Input: part model. Units: mm. Frame: model coordinates. A direction names the side the tool comes from. Round coordinates to 2 decimals unless told otherwise and drop trailing zeros. Write each loop counter-clockwise with the first axis right and the second up, starting at its lowest first coordinate (ties: lowest second). Pieces come first, ordered by that corner, then holes. Notation, with made-up numbers: M 24.5,46.5 L 76.5,46.5 A18 cw 76.5,73.5 Z; hole C 3.25,-37 d8. An arc over 180 degrees is marked long. Write each question's results on one line, items separated by ' | '. Start each with the question number.
```python
from build123d import *

# Parameters (mm, degrees)
BOSS_EXTRUDE1_DEPTH  = 4
CUT_EXTRUDE1_DEPTH   = 10
M3_CLEARANCE_HOLE3_D = 3.4
M3_CLEARANCE_HOLE4_D = 3.4


with BuildPart() as part:
    # Sketch1 → Boss-Extrude1 (new body)
    with BuildSketch(Plane(origin=(0, 0, 0), x_dir=(1, 0, 0), z_dir=(0, 1, 0))):
        with BuildLine():
            Line((-9.515488572, -74.994808418), (9.515488572, -74.994808418))
            ThreePointArc((9.515488572, -74.994808418), (13.049333225, -73.843719838), (15.227255138, -70.832122406))
            Line((15.227255138, -70.832122406), (21.674585029, -50.788926983))
            ThreePointArc((21.674585029, -50.788926983), (21.904821248, -49.783840665), (21.959569126, -48.754175722))
            Line((21.959569126, -48.754175722), (20.905492982, -16.738783097))
            ThreePointArc((20.905492982, -16.738783097), (20.516685602, -14.802919609), (19.520547525, -13.098088957))
            Line((19.520547525, -13.098088957), (13, -5.263157895))
            Line((13, -5.263157895), (13, 5.263157895))
            Line((13, 5.263157895), (19.670378922, 13.278122714))
            ThreePointArc((19.670378922, 13.278122714), (20.587655893, 14.78617896), (21.026416806, 16.495892253))
            Line((21.026416806, 16.495892253), (23.354507229, 38.891979018))
            ThreePointArc((23.354507229, 38.891979018), (23.340591043, 40.254469199), (23.019622055, 41.578686728))
            Line((23.019622055, 41.578686728), (18.764127525, 53.179369038))
            ThreePointArc((18.764127525, 53.179369038), (16.566422509, 56.032274923), (13.131169609, 57.113023201))
            Line((13.131169609, 57.113023201), (-14.108422678, 57.113023201))
            ThreePointArc((-14.108422678, 57.113023201), (-17.566572488, 56.016205829), (-19.760402704, 53.126756496))
            Line((-19.760402704, 53.126756496), (-23.659003651, 42.184485876))
            ThreePointArc((-23.659003651, 42.184485876), (-23.973087581, 40.807997325), (-23.956822357, 39.396223658))
            Line((-23.956822357, 39.396223658), (-20.971772171, 16.465578606))
            ThreePointArc((-20.971772171, 16.465578606), (-20.532623688, 14.866769408), (-19.672669362, 13.44919373))
            Line((-19.672669362, 13.44919373), (-13, 5.263157895))
            Line((-13, 5.263157895), (-13, -5.263157895))
            Line((-13, -5.263157895), (-19.456827239, -13.021524214))
            ThreePointArc((-19.456827239, -13.021524214), (-20.441610734, -14.696742104), (-20.839350394, -16.598834814))
            Line((-20.839350394, -16.598834814), (-22.202521241, -47.927982232))
            ThreePointArc((-22.202521241, -47.927982232), (-22.154511659, -48.989610746), (-21.919959446, -50.026117032))
            Line((-21.919959446, -50.026117032), (-15.227255138, -70.832122406))
            ThreePointArc((-15.227255138, -70.832122406), (-13.049333225, -73.843719838), (-9.515488572, -74.994808418))
        make_face()
    extrude(amount=BOSS_EXTRUDE1_DEPTH)

    # Sketch6 → Cut-Extrude1 (cut)
    with BuildSketch(Plane(origin=(0, 4, 0), x_dir=(1, 0, 0), z_dir=(0, 1, 0))):
        Polygon((-10.921572875, 24.5), (10.921572875, 24.5), (0, 35.421572875), align=None)
        Polygon((-7.79159133, -53.303689334), (7.79159133, -53.303689334), (0, -56.489348074), align=None)
        Polygon((-13.076324897, -55.464397842), (-13.076324897, -61.835715323), (-5.284733567, -58.650056583), align=None)
        Polygon((13.75, 27.328427125), (2.828427125, 38.25), (13.75, 49.171572875), align=None)
        Polygon((-13.5, -29.271972435), (-3.109490994, -38), (-13.5, -46.728027565), align=None)
        Polygon((-10.104794721, -49.1), (0, -40.611972435), (10.104794721, -49.1), align=None)
        Polygon((-7.79159133, -63.996423832), (7.79159133, -63.996423832), (0, -60.810765091), align=None)
        Polygon((-13.75, 27.328427125), (-2.828427125, 38.25), (-13.75, 49.171572875), align=None)
        Polygon((13.076324897, -55.464397842), (13.076324897, -61.835715323), (5.284733567, -58.650056583), align=None)
        Polygon((0, 41.078427125), (10.921572875, 52), (-10.921572875, 52), align=None)
        Polygon((-10.104794721, -26.9), (10.104794721, -26.9), (0, -35.388027565), align=None)
        Polygon((3.109490994, -38), (13.5, -29.271972435), (13.5, -46.728027565), align=None)
    extrude(amount=-CUT_EXTRUDE1_DEPTH, mode=Mode.SUBTRACT)

    # M3 Clearance Hole3 (through all)
    with Locations(Plane(origin=(0, 4, 0), x_dir=(1, 0, 0), z_dir=(0, 1, 0))):
        with Locations((7.62, -69.497474683), (-7.62, -69.497474683), (-26.177409906, -26.177409906), (26.177409906, -26.177409906), (26.177409906, 26.177409906), (-26.177409906, 26.177409906), (-15, -25.4), (-15.25, 23), (-15.25, 53.5), (15.25, 53.5), (15.25, 23), (-15, -50.6), (15, -50.6), (15, -25.4), (20, 38.25), (-20, 38.25)):
            Hole(M3_CLEARANCE_HOLE3_D / 2)

    # M3 Clearance Hole4 (through all)
    with Locations(Plane(origin=(0, 4, 0), x_dir=(1, 0, 0), z_dir=(0, 1, 0))):
        with Locations((-10.606601718, 10.606601718), (-16.263455967, 16.263455967), (10.606601718, 10.606601718), (16.263455967, 16.263455967), (16.263455967, -16.263455967), (10.606601718, -10.606601718), (-10.606601718, -10.606601718), (-16.263455967, -16.263455967)):
            Hole(M3_CLEARANCE_HOLE4_D / 2)


solid = part.part
```
1. Access query for faces 4 (the face through (-20.43, 1.97, 14.67)), 5 (the face through (-8.377, 2.028, 33.575)), 6 (the face through (16.288, 1.972, -9.215)). Directions: +Z, -Z, +X, -X, +Y, -Y. A direction counts if a zero-diameter tool reaches every point of the face in a straight line with its end or side. Return the directions, or none.
2. Draft query along Z for faces 1 (the face through (-13.092, 1.972, 73.812)), 2 (the face through (-1, 0, 8)), 3 (the face through (-13.5, 2, 38)). Return one class per face: +Z half, -Z half, draft (parallel to the pull), parting line (faces both ways), or undercut.
3. Cut plane C-C on y = 2.25. Give the number of separate pieces and of enclosed holes in the cut face, and give its area (3 significant figures).
4. Contact query for flat-ended pins moving along their axis: P1, Ø2, axis at y = 2.5, z = -0.5, coming from the +X side; P2, Ø5.5, axis at x = 15, z = 25.4, coming from the -Y side; P3, Ø2.5, axis at x = -7.62, z = 69.5, coming from the +Y side; P4, Ø1, axis at y = 3, z = 28.5, coming from the -X side. Output: stop coordinate, or through.
5. Cut plane B-B on z = 25.4. Output: boundary loops of the cut face in (x, y), and give its area (3 significant figures).
6. Line query: L1, parallel to X at y = 1.25, z = 25.4; L2, parallel to X at y = 0.8, z = -43; L3, parallel to X at y = 2.75, z = -38.25. Output: solid intervals per line, ascending. Write a range as from..to.
7. Cut plane A-A on z = -23. Output: boundary loops of the cut face in (x, y), and give its area (3 significant figures).
Answers follow:
1) face 4: -X, +Y, -Y | face 5: +Y, -Y | face 6: +X, +Y, -Y
2) face 1: +Z half | face 2: draft | face 3: undercut
3) separate pieces: 1 | enclosed holes: 32 | area: 4,040 mm2
4) P1: stops at x = 13 | P2: stops at y = 0 | P3: passes through | P4: stops at x = -21.38
5) outline: M -21.22,0 L -16.7,0 L -16.7,4 L -21.22,4 Z; M -13.3,0 L 13.3,0 L 13.3,4 L -13.3,4 Z; M 16.7,0 L 21.19,0 L 21.19,4 L 16.7,4 Z | area: 142 mm2
6) L1: x = -21.22..-16.7, -13.3..13.3, 16.7..21.19 | L2: x = -23.37..-13.75, -7.58..-1.92, 1.92..7.58, 13.75..22.5 | L3: x = -23.81..-21.7, -18.3..-13.75, -2.83..2.83, 13.75..18.3, 21.7..23.29
7) outline: M -21.82,0 L -16.95,0 L -16.95,4 L -21.82,4 Z; M -13.55,0 L 13.55,0 L 13.55,4 L -13.55,4 Z; M 16.95,0 L 21.7,0 L 21.7,4 L 16.95,4 Z | area: 147 mm2
